```python
from build123d import *

# Parameters (mm, degrees)
SKETCH1_R           = 2.5
BOSS_EXTRUDE1_DEPTH = 5
CUT_EXTRUDE1_DEPTH  = 3


with BuildPart() as part:
    # Sketch1 → Boss-Extrude1 (new body)
    with BuildSketch(Plane.XY):
        Polygon((-9.814954576, 0), (-4.907477288, -8.5), (4.907477288, -8.5), (9.814954576, 0), (4.907477288, 8.5), (-4.907477288, 8.5), align=None)
        Circle(SKETCH1_R, mode=Mode.SUBTRACT)
    extrude(amount=BOSS_EXTRUDE1_DEPTH)

    # Sketch2 → Cut-Extrude1 (cut)
    with BuildSketch(Plane.XY.offset(5)):
        Polygon((3.464101615, -6), (6.92820323, 0), (3.464101615, 6), (-3.464101615, 6), (-6.92820323, 0), (-3.464101615, -6), align=None)
    extrude(amount=-CUT_EXTRUDE1_DEPTH, mode=Mode.SUBTRACT)


solid = part.part
```
The listing builds one solid part. Answer for the finished solid, in the listing's coordinates (mm). A direction names the side the tool comes from. Give positions to 0.01 mm unless a question says otherwise; leave off trailing zeros. Write each loop counter-clockwise with the first axis right and the second up, starting at its lowest first coordinate (ties: lowest second). Pieces come first, ordered by that corner, then holes. Notation, with made-up numbers: (-6.5, -30.5) -> (-0.5, -30.5) arc R16 cw to (-0.5, -13.5) -> close; hole circle Ø1 at (-8, 71). An arc over 180 degrees is marked (long way). Write item = value, one per line. Start each with the question number.
1) The part is cut by section D-D, the plane y = 3.75. Determine the outline of the cut face in (x, z).
2) Straight lines are drawn through the part: line 1 along Y through (x, z) = (0, 3.9); line 2 along Y through (x, z) = (0, 0.6); line 3 along X through (y, z) = (4.5, 3.1). For each, find the intervals that lie inside material, in ascending order.
3) Which of the six approach directions +Z, -Z, +X, -X, +Y, -Y give full straight-line access (tool end or side, diameter ignored) to faces 1 (the face through (0, -8.5, 2)), 2 (the face through (0, 6, 4))?
4) The part is cut by section A-A, the plane x = 0. Determine the outline of the cut face in (y, z).
5) This flat-tipped pin is pushed along its axis until it touches: pin 1 (6 mm diameter, centred on x = -2, y = -1.5, fed in from +Z). Where does it stop, or does it pass through?
6) The part is cut by section C-C, the plane y = -2. Determine the outline of the cut face in (x, z).
7) Determine the mould class of faces 3 (the face through (-5.172, 3.042, 3.521)), 4 (the face through (0, 8.5, 2)), 5 (the face through (2, 2, 0)) for opening direction Y: +Y half, -Y half, draft (parallel to the pull), parting line (faces both ways), or undercut.
8) The part is cut by section B-B, the plane z = 0.9. Determine the outline of the cut face in (x, y).
Solutions:
q1.outline = (-7.65, 0) -> (7.65, 0) -> (7.65, 5) -> (4.76, 5) -> (4.76, 2) -> (-4.76, 2) -> (-4.76, 5) -> (-7.65, 5) -> close
q2.line_1 = -8.5 to -6, 6 to 8.5
q2.line_2 = -8.5 to -2.5, 2.5 to 8.5
q2.line_3 = -7.22 to -4.33, 4.33 to 7.22
q3.face_1 = +Z, -Z, +X, -X, -Y
q3.face_2 = +Z
q4.outline = (-8.5, 0) -> (-2.5, 0) -> (-2.5, 2) -> (-6, 2) -> (-6, 5) -> (-8.5, 5) -> close; (2.5, 0) -> (8.5, 0) -> (8.5, 5) -> (6, 5) -> (6, 2) -> (2.5, 2) -> close
q5.pin_1 = 2
q6.outline = (-8.66, 0) -> (-1.5, 0) -> (-1.5, 2) -> (-5.77, 2) -> (-5.77, 5) -> (-8.66, 5) -> close; (1.5, 0) -> (8.66, 0) -> (8.66, 5) -> (5.77, 5) -> (5.77, 2) -> (1.5, 2) -> close
q7.face_3 = undercut
q7.face_4 = +Y half
q7.face_5 = draft
q8.outline = (-9.81, 0) -> (-4.91, -8.5) -> (4.91, -8.5) -> (9.81, 0) -> (4.91, 8.5) -> (-4.91, 8.5) -> close; hole circle Ø5 at (0, 0)
